Geometry: see drawing. Coordinates: mm, zero at the bounding-box minimum. A direction names the side the tool comes from. Coordinates: 2 decimals unless noted, no trailing zeros. Write each loop counter-clockwise with the first axis right and the second up, starting at its lowest first coordinate (ties: lowest second). Pieces come first, ordered by that corner, then holes. Notation, with made-up numbers: (73.5, -18.5) -> (129.5, -18.5) arc R23 cw to (129.5, -0.5) -> close; hole circle Ø1 at (-4, -21.5). An arc over 180 degrees is marked (long way). Use one line per item in the form item = value. Start each with the question number.
(1) Ray query, line 1 along Y through (x, z) = (1.25, 3.5); line 2 along Z through (x, y) = (5, 12.5); line 3 along Z through (x, y) = (3.5, 4.5). Return the intervals inside material, ascending.
(2) Cut plane B-B on x = 6. Return the cut outline in (y, z).
(3) First-contact query: pin 1 (3 mm diameter, centred on y = 9.5, z = 4, fed in from -X); pin 2 (4 mm diameter, centred on x = 8, y = 10.5, fed in from +Z); pin 3 (1 mm diameter, centred on y = 8.5, z = 4, fed in from -X). Flat tips, straight axial feed; report the tip coordinate or a pass-through.
(4) Cut plane A-A on z = 6. Return the cut outline in (x, y), plus the area to 3 significant figures.
(5) Set-up query: the marked faces 1 and 2. Return all of +Z, -Z, +X, -X, +Y, -Y with unobstructed straight access to the full face (end or side cutting, diameter ignored); none if empty.
(6) Cut plane D-D on x = 9.5. Return the cut outline in (y, z).
(7) Cut plane C-C on y = 4.25. Return the cut outline in (x, z), plus the area to 3 significant figures.
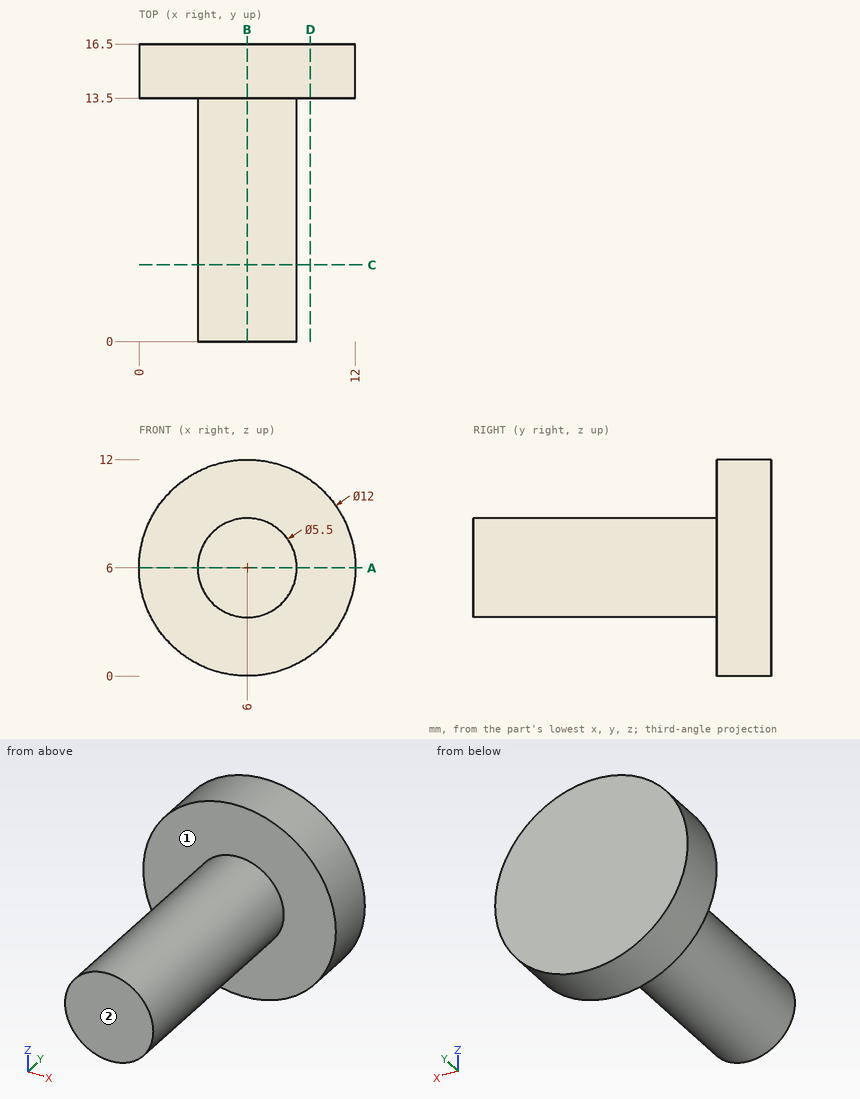
Values:
q1.line_1 = 13.5 to 16.5
q1.line_2 = 3.44 to 8.56
q1.line_3 = 4.85 to 7.15
q2.outline = (0, 3.25) -> (13.5, 3.25) -> (13.5, 0) -> (16.5, 0) -> (16.5, 12) -> (13.5, 12) -> (13.5, 8.75) -> (0, 8.75) -> close
q3.pin_1 = 3.3
q3.pin_2 = 8.75
q3.pin_3 = 3.7
q4.outline = (0, 13.5) -> (3.25, 13.5) -> (3.25, 0) -> (8.75, 0) -> (8.75, 13.5) -> (12, 13.5) -> (12, 16.5) -> (0, 16.5) -> close
q4.area = 110 mm2
q5.face_1 = -Y
q5.face_2 = +Z, -Z, +X, -X, -Y
q6.outline = (13.5, 1.13) -> (16.5, 1.13) -> (16.5, 10.87) -> (13.5, 10.87) -> close
q7.outline = circle Ø5.5 at (6, 6)
q7.area = 23.8 mm2
